```python
from build123d import *

# Parameters (mm, degrees)
FILLET_1_R          = 2
SKETCH_2_R          = 7.321356554
SKETCH_2_W          = 2
SKETCH_2_H          = 11.961651185
CUT_EXTRUDE_1_DEPTH = 8
SKETCH_3_R          = 1.5
CUT_EXTRUDE_2_DEPTH = 2
FILLET_2_R          = 0.2


with BuildPart() as part:
    # 草图1 → 旋转1 (revolve)
    with BuildSketch(Plane.XY):
        Polygon((0, 0), (0, 2.25), (-22, 2.25), (-22, 3), (-27, 3), (-27, 2.5), (-35, 2.5), (-35, 0), align=None)
    revolve(axis=Axis((0, 0, 0), (-1, 0, 0)))

    # 圆角1
    fillet_1_edges = [part.edges().sort_by_distance(p)[0] for p in [
        (-35, -2.5, 0),
    ]]
    fillet(fillet_1_edges, radius=FILLET_1_R)

    # 草图2 → 切除-拉伸1 (cut)
    with BuildSketch(Plane.ZY.offset(35)):
        Circle(SKETCH_2_R)
        with Locations((0, -0.178000761)):
            Rectangle(SKETCH_2_W, SKETCH_2_H, mode=Mode.SUBTRACT)
    extrude(amount=-CUT_EXTRUDE_1_DEPTH, mode=Mode.SUBTRACT)

    # 草图3 → 切除-拉伸2 (cut)
    with BuildSketch(Plane(origin=(0, 0, -1), x_dir=(-1, 0, 0), z_dir=(0, 0, -1))):
        with Locations(Location((31.5, 0, 0), (0, 0, 90))):
            Circle(SKETCH_3_R)
    extrude(amount=-CUT_EXTRUDE_2_DEPTH, mode=Mode.SUBTRACT)

    # 圆角2
    fillet_2_edges = [part.edges().sort_by_distance(p)[0] for p in [
        (-27, -3, 0),
        (-22, -3, 0),
        (0, -2.25, 0),
    ]]
    fillet(fillet_2_edges, radius=FILLET_2_R)


solid = part.part
```
Source: CAD feature listing. Evaluate the final solid. Frame: model axes, mm. A direction names the side the tool comes from. Coordinates: 2 decimals unless noted, no trailing zeros. Loops run counter-clockwise (first coordinate to the right, second up) from the corner with the lowest first, then second, coordinate; pieces in that order, holes last. Notation, with made-up numbers: M 81.25,36 L 123.25,36 A18 ccw 123.25,60 Z; hole C -31.5,6.25 d4. An arc over 180 degrees is marked long. Use CSV: the item, a comma, the result in double quotes.
(1) Reachability of faces 1 (the face through (-30, 2.5, 0)), 2 (the face through (-30, -2.5, 0)), 3 (the face through (-11.25, -0.29, -2.23)), 4 (the face through (-30, -1, 1)), 5 (the face through (-30, 1, -1)) from +Z, -Z, +X, -X, +Y, -Y: full face, straight path, thin tool, end or side. Return the list, or none.
Answers follow:
face 1,"-X, +Y"
face 2,"-X, -Y"
face 3,"+X"
face 4,"+Z, -X, +Y, -Y"
face 5,"-Z, -X, +Y, -Y"
(2) Cut plane A-A on x = -31.5. Return loops of the section in (y, z).
Answers follow:
outline,"M -2.29,-1 L -1.5,-1 L -1.5,1 L -2.29,1 A2.5 ccw Z; M 1.5,-1 L 2.29,-1 A2.5 ccw 2.29,1 L 1.5,1 Z"
(3) Line query: line 1 (X direction, y = 0, z = -0.2); line 2 (X direction, y = 2, z = -2); line 3 (Z direction, x = -29.5, y = -1.75). Output: solid intervals per line, ascending. Write a range as [from, to].
Answers follow:
line 1,"[-35, -33], [-30, 0]"
line 2,"[-27, -22]"
line 3,"[-1, 1]"
(4) Contact query for flat-ended pins moving along their axis: pin 1 (3.5 mm diameter, centred on x = -30.5, y = 1, fed in from -Z); pin 2 (1.4 mm diameter, centred on x = -29.5, y = -0.5, fed in from +Z); pin 3 (1 mm diameter, centred on x = -5.5, z = -1.5, fed in from +Y). Output: stop coordinate, or through.
Answers follow:
pin 1,"z = -1"
pin 2,"z = 1"
pin 3,"y = 2.02"
